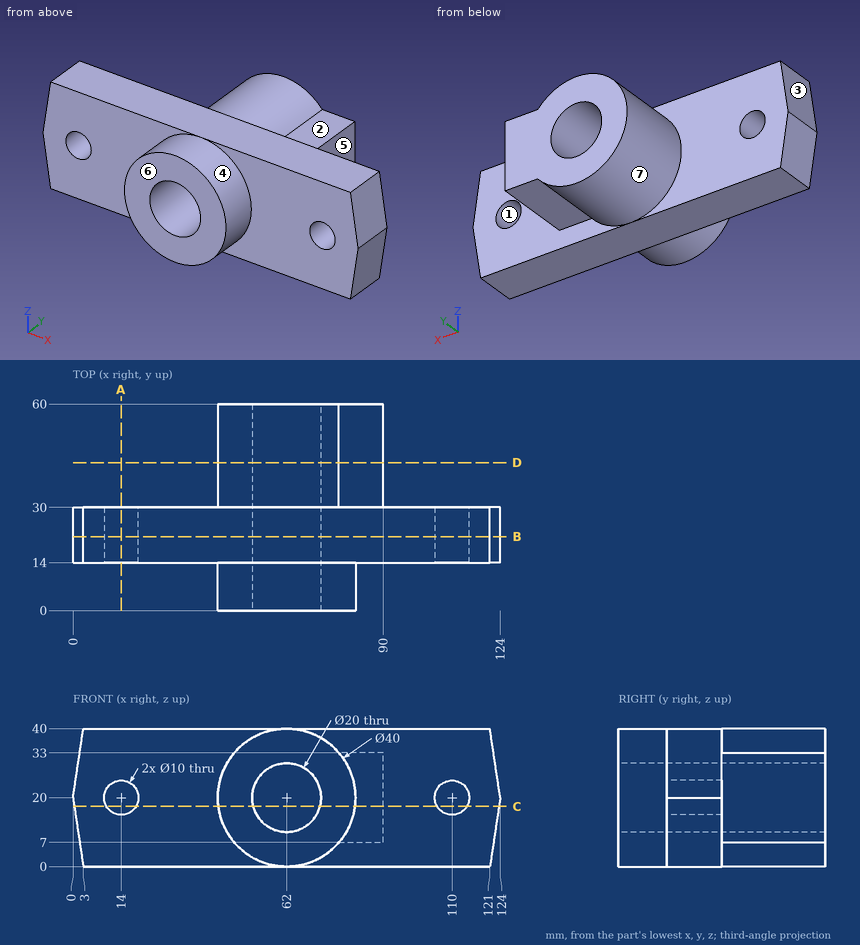
Here's the drawing with two shaded views (mm, measured from the low corner). I have some questions. A direction names the side the tool comes from. Give positions to 0.01 mm unless a question says otherwise; leave off trailing zeros. Loops run counter-clockwise (first coordinate to the right, second up) from the corner with the lowest first, then second, coordinate; pieces in that order, holes last. Notation, with made-up numbers: M 78,37 L 129,37 A17 cw 129,41 Z; hole C -6.75,22.5 d7. An arc over 180 degrees is marked long. Answer in a Markdown table with one row per item.
1. Suppose I cut it at A-A on x = 14. Write out the boundary of the cut face in (y, z).
Taken from the geometry:
| item | result |
|---|---|
| outline | M 14,0 L 30,0 L 30,15 L 14,15 Z; M 14,25 L 30,25 L 30,40 L 14,40 Z |
2. Suppose I cut it at D-D on y = 43. Write out the boundary of the cut face in (x, z).
Taken from the geometry:
| item | result |
|---|---|
| outline | M 77.2,7 L 90,7 L 90,33 L 77.2,33 A20 ccw long Z; hole C 62,20 d20 |
3. Suppose I cut it at B-B on y = 21.5. Write out the boundary of the cut face in (x, z), plus the area to 3 significant figures.
Taken from the geometry:
| item | result |
|---|---|
| outline | M 0,20 L 3,0 L 121,0 L 124,20 L 121,40 L 3,40 Z; hole C 14,20 d10; hole C 62,20 d20; hole C 110,20 d10 |
| area | 4,370 mm² |
4. Suppose I cut it at C-C on z = 17.5. Write out the boundary of the cut face in (x, y) (3 decimals), plus the area to 3 significant figures.
Taken from the geometry:
| item | result |
|---|---|
| outline | M 0.375,14 L 9.67,14 L 9.67,30 L 0.375,30 Z; M 18.33,14 L 42.157,14 L 42.157,0 L 52.318,0 L 52.318,60 L 42.157,60 L 42.157,30 L 18.33,30 Z; M 71.682,0 L 81.843,0 L 81.843,14 L 105.67,14 L 105.67,30 L 90,30 L 90,60 L 71.682,60 Z; M 114.33,14 L 123.625,14 L 123.625,30 L 114.33,30 Z |
| area | 2,520 mm² |
5. Which directions (+Z, -Z, +X, -X, +Y, -Y) give clear straight access to the entire face, cutting with the end or side of a thin tool? Please do the marked faces 5, 6 and 7.
Taken from the geometry:
| item | result |
|---|---|
| face 5 | +Z, -Z, +X, +Y |
| face 6 | +Z, -Z, +X, -X, -Y |
| face 7 | +Y |
6. Thinking about a two-plate mould opening in X: for the marked faces 1, 2, 3 and 4, which applies, released by +X, released by -X, zero draft, split by the parting line, or undercut?
Taken from the geometry:
| item | result |
|---|---|
| face 1 | undercut |
| face 2 | zero draft |
| face 3 | released by -X |
| face 4 | split by the parting line |
7. For pin 1 Ø21 at (y, z) = (45.5, 23.5) entering from +X; pin 2 Ø11.5 at (x, z) = (14, 20) entering from -Y; pin 3 Ø2 at (y, z) = (35.5, 22) entering from -X (3 decimals), each with a flat end and sliding along its axis, tell me the tip position at first contact or that it passes through.
Taken from the geometry:
| item | result |
|---|---|
| pin 1 | stops at x = 90 |
| pin 2 | stops at y = 14 |
| pin 3 | stops at x = 42.025 |
8. If I drill on line 1 along X through (y, z) = (22.75, 20); line 2 along Z through (x, y) = (14, 25); line 3 along Z through (x, y) = (62, 36.5), over which ranges is the centre line in solid material (lowest first)?
Taken from the geometry:
| item | result |
|---|---|
| line 1 | x = 0 to 9, 19 to 52, 72 to 105, 115 to 124 |
| line 2 | z = 0 to 15, 25 to 40 |
| line 3 | z = 0 to 10, 30 to 40 |
